The model under review builds one solid part; all positions refer to its coordinate system, in mm. A direction names the side the tool comes from. Round coordinates to 2 decimals unless told otherwise and drop trailing zeros. Write each loop counter-clockwise with the first axis right and the second up, starting at its lowest first coordinate (ties: lowest second). Pieces come first, ordered by that corner, then holes. Notation, with made-up numbers: (27, -32) -> (66, -32) arc R34 cw to (66, 5) -> close; hole circle Ø7 at (2, -1.5). An arc over 180 degrees is marked (long way). Return JSON: item names as keys, results as strings. Group by question number.
1. For line 1 along X through (y, z) = (0.85, 1.55); line 2 along Z through (x, y) = (0, 1.45), list the stretches that pass through material, from the lowest coordinate up. Write a range as from..to.
2. Clearance check with flat-ended pins moving along their axes: P1, Ø1.6, axis at y = -0.5, z = 2, coming from the +X side; P2, Ø0.8, axis at y = 0, z = 1.5, coming from the -X side. State where each tip first meets the part, or that it passes through.
3. Tool access review of faces 1 (the flat face through (-4.15, 0, 2)), 2 (the flat face through (4.15, 0, 2)), 3 (the flat face through (0, -1.75, 1)): name each direction out of +Z, -Z, +X, -X, +Y, -Y from which nothing blocks a thin tool from reaching the whole face with its end or side.
4. Take a section at D-D, the plane y = 1.4. Write out the cut boundary in (x, z).
5. Take a section at C-C, the plane x = 4.25. Write out the cut boundary in (y, z).
6. Take a section at A-A, the plane y = -0.3. Write out the cut boundary in (x, z), then the cut area to 3 significant figures.
7. Take a section at B-B, the plane z = 2.05. Write out the cut boundary in (x, y), then the cut area to 4 significant figures.
from build123d import *

# Parameters (mm, degrees)
SKETCH_1_W      = 9.8
SKETCH_1_H      = 3.5
EXTRUDE_1_DEPTH = 1
SKETCH_2_W      = 8.3
SKETCH_2_H      = 3.5
EXTRUDE_2_DEPTH = 2
FILLET_2_R      = 0.5


with BuildPart() as part:
    # 草图1 → 凸台-拉伸1 (new body)
    with BuildSketch(Plane.XY):
        Rectangle(SKETCH_1_W, SKETCH_1_H)
    extrude(amount=EXTRUDE_1_DEPTH)

    # 草图2 → 凸台-拉伸2 (add)
    with BuildSketch(Plane.XY.offset(1)):
        Rectangle(SKETCH_2_W, SKETCH_2_H)
    extrude(amount=EXTRUDE_2_DEPTH)

    # 圆角2
    fillet_2_edges = [part.edges().sort_by_distance(p)[0] for p in [
        (4.15, 0, 3),
        (0, 1.75, 3),
        (-4.15, 0, 3),
        (0, -1.75, 3),
    ]]
    fillet(fillet_2_edges, radius=FILLET_2_R)


solid = part.part
Output:
{
 "1": {"line 1": "x = -4.15..4.15", "line 2": "z = 0..2.96"},
 "2": {"P1": "stops at x = 4.15", "P2": "stops at x = -4.15"},
 "3": {"face 1": "+Z, -X, +Y, -Y", "face 2": "+Z, +X, +Y, -Y", "face 3": "+Z, -Z, +X, -X, -Y"},
 "4": {"outline": "(-4.9, 0) -> (4.9, 0) -> (4.9, 1) -> (4.15, 1) -> (4.15, 2.5) arc R0.5 ccw to (3.8, 2.98) -> (-3.8, 2.98) arc R0.5 ccw to (-4.15, 2.5) -> (-4.15, 1) -> (-4.9, 1) -> close"},
 "5": {"outline": "(-1.75, 0) -> (1.75, 0) -> (1.75, 1) -> (-1.75, 1) -> close"},
 "6": {"outline": "(-4.9, 0) -> (4.9, 0) -> (4.9, 1) -> (4.15, 1) -> (4.15, 2.5) arc R0.5 ccw to (3.65, 3) -> (-3.65, 3) arc R0.5 ccw to (-4.15, 2.5) -> (-4.15, 1) -> (-4.9, 1) -> close", "area": "26.3 mm^2"},
 "7": {"outline": "(-4.15, -1.75) -> (4.15, -1.75) -> (4.15, 1.75) -> (-4.15, 1.75) -> close", "area": "29.05 mm^2"}
}
